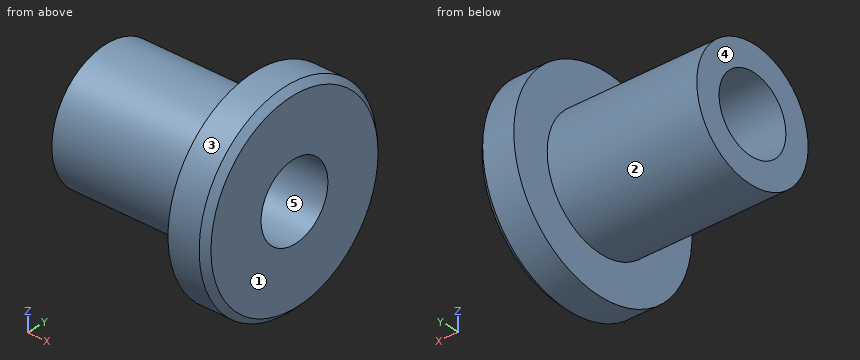
```python
from build123d import *

# Parameters (mm, degrees)
HOLE_WIZARD_6_0_6_1_D     = 6
HOLE_WIZARD_6_0_6_1_DEPTH = 18.197418143
HOLE_WIZARD_6_0_6_1_TIP   = 1.802581857
CHAMFER_1_SIZE            = 0.5


with BuildPart() as part:
    # 草图1 → 旋转1 (revolve)
    with BuildSketch(Plane.XY):
        Polygon((-9.428571429, 0), (-9.428571429, 5), (2.571428571, 5), (2.571428571, 8), (5.571428571, 8), (5.571428571, 0), align=None)
    revolve(axis=Axis((5.571428571, 0, 0), (-1, 0, 0)))

    # Ø6.0 (6) 直径孔1
    with Locations(Plane.ZY.offset(9.428571429)):
        with Locations((0, 0)):
            Hole(HOLE_WIZARD_6_0_6_1_D / 2, depth=HOLE_WIZARD_6_0_6_1_DEPTH)
            with Locations((0, 0, -(HOLE_WIZARD_6_0_6_1_DEPTH + HOLE_WIZARD_6_0_6_1_TIP / 2))):  # 118° drill point
                Cone(0, HOLE_WIZARD_6_0_6_1_D / 2, HOLE_WIZARD_6_0_6_1_TIP, mode=Mode.SUBTRACT)

    # 倒角1
    chamfer_1_edges = [part.edges().sort_by_distance(p)[0] for p in [
        (5.571428571, -8, 0),
    ]]
    chamfer(chamfer_1_edges, length=CHAMFER_1_SIZE)


solid = part.part
```
Design review of the part built by this model. Coordinates are the model's own, in mm. Face numbers are marked on the shaded views. A direction names the side the tool comes from. Give positions to 0.01 mm unless a question says otherwise; leave off trailing zeros. Order: outer loops, then holes, each group sorted by start corner. A loop starts at its lowest first (then second) coordinate and runs counter-clockwise, first axis right, second up. Notation, with made-up numbers: M -20,51.5 L 13,51.5 A14 cw 13,62.5 Z; hole C 49.25,56 d1. An arc over 180 degrees is marked long. One line per question, with ' | ' between items. Start each with the question number.
Q1. The part is to be moulded in two halves that separate along Y. For the marked faces 3, 4 and 5, say which applies: +Y half, -Y half, draft (parallel to the pull), parting line (faces both ways), or undercut.
Q2. For pin 1 Ø6 at (x, z) = (-2.5, 1) entering from +Y; pin 2 Ø1 at (x, y) = (1, 1) entering from +Z; pin 3 Ø5.5 at (y, z) = (0, 0) entering from +X; pin 4 Ø1 at (x, y) = (0.5, 4.5) entering from +Z, all flat-tipped, find the tip position at first contact; note any pin that passes through.
Q3. For L1, parallel to Y at x = 0, z = 0; L2, parallel to Y at x = -5, z = 0.75; L3, parallel to Z at x = -5.75, y = 4, list the stretches that pass through material, from the lowest coordinate up. Write a range as [from, to].
Q4. We need section A-A (y = 0). Write out the cut boundary in (x, z).
Q5. We need section C-C (x = -5.25). Write out the cut boundary in (y, z).
Q6. Machinability: for the marked faces 1 and 2, which of the approach directions +Z, -Z, +X, -X, +Y, -Y give a long, thin tool a straight path to every point of the face, cutting with its end or side? Answer none if there is none.
Returned:
1) face 3: parting line | face 4: draft | face 5: undercut
2) pin 1: y = 5 | pin 2: z = 4.97 | pin 3: through | pin 4: z = 3
3) L1: [-5, -3], [3, 5] | L2: [-4.94, -2.9], [2.9, 4.94] | L3: [-3, 3]
4) outline: M -9.43,-5 L 2.57,-5 L 2.57,-8 L 5.07,-8 L 5.57,-7.5 L 5.57,-3 L -9.43,-3 Z; M -9.43,3 L 5.57,3 L 5.57,7.5 L 5.07,8 L 2.57,8 L 2.57,5 L -9.43,5 Z
5) outline: C 0,0 d10; hole C 0,0 d6
6) face 1: +Z, -Z, +X, +Y, -Y | face 2: -X
